```python
from build123d import *

# Parameters (mm, degrees)
SKETCH1_R            = 33
SKETCH1_R_2          = 17.5
SKETCH1_W            = 10.1
SKETCH1_H            = 10.1
BOSS_EXTRUDE1_DEPTH  = 90
CUT_EXTRUDE1_START   = -91
CUT_EXTRUDE1_DEPTH   = 92
MIRROR2_START        = -91
MIRROR2_COPY_1_DEPTH = 92


with BuildPart() as part:
    # Sketch1 → Boss-Extrude1 (new body)
    with BuildSketch(Plane.XY):
        Circle(SKETCH1_R)
        Circle(SKETCH1_R_2, mode=Mode.SUBTRACT)
        Polygon((15.185219507, 10.901571711), (20.235219507, 19.648428289), (28.982076086, 14.598428289), (23.932076086, 5.851571711), align=None, mode=Mode.SUBTRACT)
        with Locations((25.5, 0)):
            Rectangle(SKETCH1_W, SKETCH1_H, mode=Mode.SUBTRACT)
        Polygon((5.851571711, 23.932076086), (14.598428289, 28.982076086), (19.648428289, 20.235219507), (10.901571711, 15.185219507), align=None, mode=Mode.SUBTRACT)
        with Locations((0, 25.5)):
            Rectangle(SKETCH1_W, SKETCH1_H, mode=Mode.SUBTRACT)
        with Locations((-25.5, 0)):
            Rectangle(SKETCH1_W, SKETCH1_H, mode=Mode.SUBTRACT)
        Polygon((-23.932076086, 5.851571711), (-28.982076086, 14.598428289), (-20.235219507, 19.648428289), (-15.185219507, 10.901571711), align=None, mode=Mode.SUBTRACT)
        Polygon((-10.901571711, 15.185219507), (-19.648428289, 20.235219507), (-14.598428289, 28.982076086), (-5.851571711, 23.932076086), align=None, mode=Mode.SUBTRACT)
        Polygon((23.932076086, -5.851571711), (28.982076086, -14.598428289), (20.235219507, -19.648428289), (15.185219507, -10.901571711), align=None, mode=Mode.SUBTRACT)
        Polygon((10.901571711, -15.185219507), (19.648428289, -20.235219507), (14.598428289, -28.982076086), (5.851571711, -23.932076086), align=None, mode=Mode.SUBTRACT)
        with Locations((0, -25.5)):
            Rectangle(SKETCH1_W, SKETCH1_H, mode=Mode.SUBTRACT)
        Polygon((-5.851571711, -23.932076086), (-10.901571711, -15.185219507), (-19.648428289, -20.235219507), (-14.598428289, -28.982076086), align=None, mode=Mode.SUBTRACT)
        Polygon((-15.185219507, -10.901571711), (-23.932076086, -5.851571711), (-28.982076086, -14.598428289), (-20.235219507, -19.648428289), align=None, mode=Mode.SUBTRACT)
    extrude(amount=BOSS_EXTRUDE1_DEPTH)

    # Sketch2 → Cut-Extrude1 (cut)
    with BuildSketch(Plane.XY.offset(90).offset(CUT_EXTRUDE1_START)):
        with BuildLine():
            Line((-195.710732602, 14.035729655), (-27.032017462, 18.9280224))
            ThreePointArc((-27.032017462, 18.9280224), (-21.370045373, 21.370045373), (-18.9280224, 27.032017462))
            Line((-18.9280224, 27.032017462), (-14.035729655, 195.710732602))
            Line((-14.035729655, 195.710732602), (-252.683769537, 434.358772484))
            Line((-252.683769537, 434.358772484), (-434.358772484, 252.683769537))
            Line((-434.358772484, 252.683769537), (-195.710732602, 14.035729655))
        make_face()
    cut_extrude1 = extrude(amount=CUT_EXTRUDE1_DEPTH, mode=Mode.SUBTRACT)

    # Mirror1: Cut-Extrude1 across plane
    add(cut_extrude1.mirror(Plane(origin=(0, 0, 0), x_dir=(0, 0, 1), z_dir=(1, 0, 0))), mode=Mode.SUBTRACT)

    # Mirror2: Cut-Extrude1 across plane
    add(cut_extrude1.mirror(Plane.ZX), mode=Mode.SUBTRACT)

    # Mirror2 copy 1 sketch → Mirror2 copy 1 (cut)
    with BuildSketch(Plane(origin=(0, 0, 90), x_dir=(-1, 0, 0), z_dir=(0, 0, 1)).offset(MIRROR2_START)):
        with BuildLine():
            Line((-195.710732602, 14.035729655), (-27.032017462, 18.9280224))
            ThreePointArc((-27.032017462, 18.9280224), (-21.370045373, 21.370045373), (-18.9280224, 27.032017462))
            Line((-18.9280224, 27.032017462), (-14.035729655, 195.710732602))
            Line((-14.035729655, 195.710732602), (-252.683769537, 434.358772484))
            Line((-252.683769537, 434.358772484), (-434.358772484, 252.683769537))
            Line((-434.358772484, 252.683769537), (-195.710732602, 14.035729655))
        make_face()
    extrude(amount=MIRROR2_COPY_1_DEPTH, mode=Mode.SUBTRACT)


solid = part.part
```
For this review, take the finished solid that the model builds, in its own axes (mm). A direction names the side the tool comes from. Round coordinates to 2 decimals unless told otherwise and drop trailing zeros. Loops run counter-clockwise (first coordinate to the right, second up) from the corner with the lowest first, then second, coordinate; pieces in that order, holes last.
Q1. Mouldability with a two-part tool opening along X and no side actions: class faces 3 (the face through (33, 0, 44)), 4 (the face through (17.75, -15.34, 44.37)), 5 (the face through (-5.05, -26, 44)), 6 (the face through (-21.43, -21.31, 44.37)) as +X half, -X half, draft (parallel to the pull), parting line (faces both ways), or undercut.
Result sheet:
face 3: +X half
face 4: undercut
face 5: undercut
face 6: -X half
Q2. Add section C-C on z = 35. Give the number of separate pieces and of enclosed holes in the cut face, plus the area to 3 significant figures.
Result sheet:
separate pieces: 1
enclosed holes: 13
area: 1,150 mm2
Q3. Insertion check: pin 1 Ø8 at (y, z) = (-0.5, 63) entering from +X; pin 2 Ø5 at (y, z) = (-23.5, 48.5) entering from +X; pin 3 Ø6 at (x, z) = (-16, 33.5) entering from +Y. Each pin has a flat end and moves straight along its axis. Give the tip position at first contact, or say it passes through.
Result sheet:
pin 1: stops at x = 33
pin 2: stops at x = 21.76
pin 3: stops at y = 30.33
Q4. Add section A-A on x = 0. Write out the cut boundary in (y, z).
Result sheet:
outline: (-33, 0) - (-30.55, 0) - (-30.55, 90) - (-33, 90) - close; (-20.45, 0) - (-17.5, 0) - (-17.5, 90) - (-20.45, 90) - close; (17.5, 0) - (20.45, 0) - (20.45, 90) - (17.5, 90) - close; (30.55, 0) - (33, 0) - (33, 90) - (30.55, 90) - close
Q5. Machinability: for faces 1 (the face through (-8.34, -19.62, 44.37)), 2 (the face through (-33, 0, 44)), which of the approach directions +Z, -Z, +X, -X, +Y, -Y give a long, thin tool a straight path to every point of the face, cutting with its end or side? Answer none if there is none.
Result sheet:
face 1: +Z, -Z
face 2: +Z, -Z, -X
Q6. To check wall thickness, follow line 1 along Y through (x, z) = (0, 69); line 2 along X through (y, z) = (-18.5, 54.5); line 3 along Y through (x, z) = (4, 48). State the ranges of each line that lie inside material, in increasing order.
Result sheet:
line 1: y = -33 to -30.55, -20.45 to -17.5, 17.5 to 20.45, 30.55 to 33
line 2: x = -27.33 to -22.22, -19.57 to -16.64, -8.99 to 8.99, 16.64 to 19.57, 22.22 to 27.33
line 3: y = -32.76 to -30.55, -20.45 to -17.04, 17.04 to 20.45, 30.55 to 32.76
